Autodesk Inventor part; units mm, degrees
ref_plane "YZ Plane" through (0, 0, 0) normal (1, 0, 0) x (0, 1, 0)
ref_plane "XZ Plane" through (0, 0, 0) normal (0, 1, 0) x (-1, 0, 0)
ref_plane "XY Plane" through (0, 0, 0) normal (0, 0, 1) x (1, 0, 0)
sketch "Sketch1" plane through (0, 0, 0) normal (0, 0, 1) x (1, 0, 0)
  circle A0 centre (0, 0) radius 7
  circle A1 centre (0, 0) radius 16
  circle A2 centre (-12.5, 0) radius 2
  circle A3 centre (0, -12.5) radius 2
  circle A4 centre (12.5, 0) radius 2
  circle A5 centre (0, 12.5) radius 2
  circle A6 centre (0, 0) radius 8
  line L0 (0, 0) -> (-12.5, 0)
  point P0 (-7, 0)
  point P1 (-7.7857, 1.8392)
  dimension "d0" = 14
  dimension "d8" = 16
  dimension "d1" = 32
  dimension "d2" = 4
  dimension "d5" = 360
  dimension "d15" = 12.5
extrude "Extrusion1" add sketch "Sketch1" along normal blind 2 contours A1
extrude "Extrusion2" add sketch "Sketch1" against normal blind 3 contours A6
extrude "Extrusion3" add sketch "Sketch1" along normal blind 2 contours A6
fillet "Fillet2" radius 0.5 1 edges at (-8, 0, 0)
properties part number "flange"
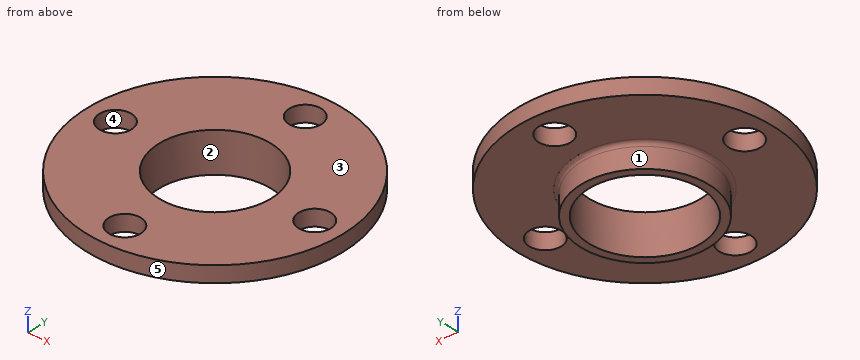
Geometry: final body of the model. Coordinates: model frame, mm. Face numbers are marked on the shaded views. A direction names the side the tool comes from. Round coordinates to 2 decimals unless told otherwise and drop trailing zeros. Order: outer loops, then holes, each group sorted by start corner. A loop starts at its lowest first (then second) coordinate and runs counter-clockwise, first axis right, second up. Notation, with made-up numbers: (2.5, -31.75) -> (31.5, -31.75) arc R13 cw to (31.5, -12.75) -> close; hole circle Ø2 at (0, 88.5). An arc over 180 degrees is marked (long way). Use one line per item in the form item = value. Start each with the question number.
1. Line query: probe 1 along Y at (x, z) = (0, 1); probe 2 along X at (y, z) = (-1, 0.6); probe 3 along X at (y, z) = (5, -2.65) (3 decimals). Output: solid intervals per line, ascending.
2. Cut plane A-A (y = 0). Return the cut outline in (x, z).
3. Draft query along X for the marked faces 3, 4 and 5. Return one class per face: pulls with the +X half, pulls with the -X half, needs draft (parallel to the pull), parting line crosses it, or undercut.
4. Cut plane C-C (x = -12.5). Return the cut outline in (y, z).
5. Reachability of the marked faces 1 and 2 from +Z, -Z, +X, -X, +Y, -Y: full face, straight path, thin tool, end or side. Return the list, or none.
6. Cut plane D-D (z = 0.55). Return the cut outline in (x, y).
7. Pin query (flat end, axial travel): pin 1 Ø3.5 at (x, y) = (0, 12.5) entering from -Z; pin 2 Ø3 at (x, y) = (1.5, -12) entering from -Z; pin 3 Ø3 at (x, z) = (8, 0.5) entering from -Y. Return the tip coordinate at first contact, or that it passes through.
Solution:
q1.probe_1 = -16 to -14.5, -10.5 to -7, 7 to 10.5, 14.5 to 16
q1.probe_2 = -15.97 to -14.23, -10.77 to -6.93, 6.93 to 10.77, 14.23 to 15.97
q1.probe_3 = -6.245 to -4.899, 4.899 to 6.245
q2.outline = (-16, 0) -> (-14.5, 0) -> (-14.5, 2) -> (-16, 2) -> close; (-10.5, 0) -> (-8.5, 0) arc R0.5 cw to (-8, -0.5) -> (-8, -3) -> (-7, -3) -> (-7, 2) -> (-10.5, 2) -> close; (7, -3) -> (8, -3) -> (8, -0.5) arc R0.5 cw to (8.5, 0) -> (10.5, 0) -> (10.5, 2) -> (7, 2) -> close; (14.5, 0) -> (16, 0) -> (16, 2) -> (14.5, 2) -> close
q3.face_3 = needs draft
q3.face_4 = undercut
q3.face_5 = parting line crosses it
q4.outline = (-9.99, 0) -> (-2, 0) -> (-2, 2) -> (-9.99, 2) -> close; (2, 0) -> (9.99, 0) -> (9.99, 2) -> (2, 2) -> close
q5.face_1 = -Z
q5.face_2 = +Z, -Z
q6.outline = circle Ø32 at (0, 0); hole circle Ø4 at (-12.5, 0); hole circle Ø14 at (0, 0); hole circle Ø4 at (0, -12.5); hole circle Ø4 at (0, 12.5); hole circle Ø4 at (12.5, 0)
q7.pin_1 = through
q7.pin_2 = 0
q7.pin_3 = -14.62
